For this review, take the finished solid that the model builds, in its own axes (mm). Round coordinates to 2 decimals unless told otherwise and drop trailing zeros. Loops run counter-clockwise (first coordinate to the right, second up) from the corner with the lowest first, then second, coordinate; pieces in that order, holes last. Notation, with made-up numbers: (-36, 52.5) -> (-19, 52.5) arc R30 cw to (-19, 77.5) -> close; hole circle Ø6 at (70, 75.25). An arc over 180 degrees is marked (long way). One line per question, with ' | ' between items. Start each with the question number.
1. Consider section A-A (y = -0.75). Count the separate pieces of the cut face and the enclosed holes in it, and give its area (3 significant figures).
2. Wall thickness on line 1 along Z through (x, y) = (28.5, -0.85) (3 decimals); line 2 along X through (y, z) = (-0.55, 141) (3 decimals); line 3 along X through (y, z) = (-0.7, 170.5): over which ranges is each line inside the solid? List them lowest first.
3. For pin 1 Ø0.5 at (x, y) = (268.5, -0.5) entering from +Z (3 decimals), flat-tipped, find the tip position at first contact; note if it passes through.
4. Consider section B-B (x = 71). Write out the cut boundary in (y, z) (1 decimal).
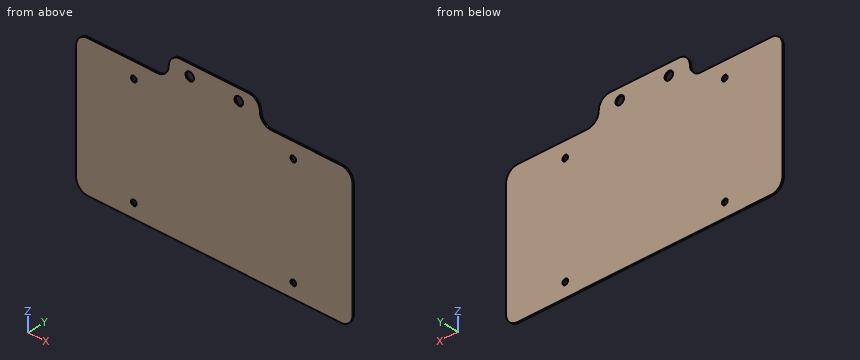
```python
from build123d import *

# Parameters (mm, degrees)
F0_R     = 3.175
F0_R_2   = 4.7625
F1_DEPTH = 1.7145


with BuildPart() as f1:
    # F0 (on Front) → F1 (new body)
    with BuildSketch(Plane.XZ):
        with BuildLine():
            ThreePointArc((0, 12.7), (3.719744, 3.719744), (12.7, 0))
            Line((12.7, 0), (295.275, 0))
            ThreePointArc((295.275, 0), (304.255256, 3.719744), (307.975, 12.7))
            Line((307.975, 12.7), (307.975, 142.875))
            ThreePointArc((307.975, 142.875), (304.255256, 151.855256), (295.275, 155.575))
            Line((295.275, 155.575), (217.4875, 155.575))
            ThreePointArc((217.4875, 155.575), (208.507244, 159.294744), (204.7875, 168.275))
            ThreePointArc((204.7875, 168.275), (201.067756, 177.255256), (192.0875, 180.975))
            Line((192.0875, 180.975), (115.8875, 180.975))
            ThreePointArc((115.8875, 180.975), (106.907244, 177.255256), (103.1875, 168.275))
            ThreePointArc((103.1875, 168.275), (99.467756, 159.294744), (90.4875, 155.575))
            Line((90.4875, 155.575), (12.7, 155.575))
            ThreePointArc((12.7, 155.575), (3.719744, 151.855256), (0, 142.875))
            Line((0, 142.875), (0, 12.7))
        make_face()
        with Locations((64.29375, 15.875)):
            Circle(F0_R, mode=Mode.SUBTRACT)
        with Locations((242.09375, 15.875)):
            Circle(F0_R, mode=Mode.SUBTRACT)
        with Locations((64.29375, 138.1125)):
            Circle(F0_R, mode=Mode.SUBTRACT)
        with Locations((126.602998, 168.275)):
            Circle(F0_R_2, mode=Mode.SUBTRACT)
        with Locations((181.371748, 168.275)):
            Circle(F0_R_2, mode=Mode.SUBTRACT)
        with Locations((242.09375, 138.1125)):
            Circle(F0_R, mode=Mode.SUBTRACT)
    extrude(amount=F1_DEPTH)


solid = f1.part
```
Answer block:
1) separate pieces: 1 | enclosed holes: 6 | area: 50,100 mm2
2) line 1: z = 0 to 155.575 | line 2: x = 0 to 62.974, 65.614 to 240.774, 243.414 to 307.975 | line 3: x = 103.38 to 122.39, 130.81 to 177.16, 185.58 to 204.59
3) pin 1: stops at z = 155.575
4) outline: (-1.7, 0) -> (0, 0) -> (0, 155.6) -> (-1.7, 155.6) -> close
